Answer from the drawing. Dimensions are ordinates in mm from the lowest x, y and z of the part. Give positions to 0.01 mm unless a question says otherwise; leave off trailing zeros. Loops run counter-clockwise (first coordinate to the right, second up) from the corner with the lowest first, then second, coordinate; pieces in that order, holes last. Notation, with made-up numbers: M 46,9.25 L 89,9.25 A25 cw 89,40.25 Z; hole C 85,82.5 d10. An arc over 180 degrees is marked long. Use a Markdown table: item, result.
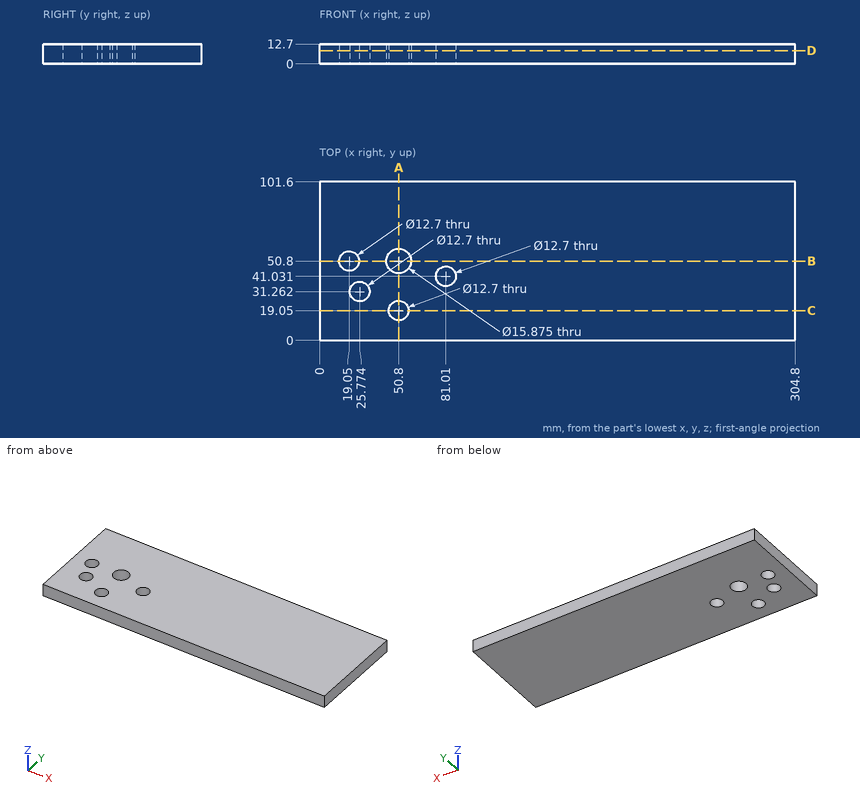
(1) A cutting plane is placed at A-A (x = 50.8). Write down the section's boundary in (y, z).
Entries:
| item | result |
|---|---|
| outline | M 0,0 L 12.7,0 L 12.7,12.7 L 0,12.7 Z; M 25.4,0 L 42.86,0 L 42.86,12.7 L 25.4,12.7 Z; M 58.74,0 L 101.6,0 L 101.6,12.7 L 58.74,12.7 Z |
(2) A cutting plane is placed at B-B (y = 50.8). Write down the section's boundary in (x, z), and give its area (3 significant figures).
Entries:
| item | result |
|---|---|
| outline | M 0,0 L 12.7,0 L 12.7,12.7 L 0,12.7 Z; M 25.4,0 L 42.86,0 L 42.86,12.7 L 25.4,12.7 Z; M 58.74,0 L 304.8,0 L 304.8,12.7 L 58.74,12.7 Z |
| area | 3,510 mm² |
(3) Consider probe 1 along Y at (x, z) = (50.8, 3.5); probe 2 along X at (y, z) = (53, 11.75) (1 decimal); probe 3 along Y at (x, z) = (19.05, 4.75). Determine where each line is inside the solid, lowest interval first. Write a range as [from, to].
Entries:
| item | result |
|---|---|
| probe 1 | y = [0, 12.7], [25.4, 42.86], [58.74, 101.6] |
| probe 2 | x = [0, 13.1], [25, 43.2], [58.4, 304.8] |
| probe 3 | y = [0, 44.45], [57.15, 101.6] |
(4) A cutting plane is placed at D-D (z = 8.5). Count the separate pieces of the cut face and the enclosed holes in it, and give its area (3 significant figures).
Entries:
| item | result |
|---|---|
| separate pieces | 1 |
| enclosed holes | 5 |
| area | 30,300 mm² |
(5) A cutting plane is placed at C-C (y = 19.05). Write down the section's boundary in (x, z), and give its area (3 significant figures).
Entries:
| item | result |
|---|---|
| outline | M 0,0 L 44.45,0 L 44.45,12.7 L 0,12.7 Z; M 57.15,0 L 304.8,0 L 304.8,12.7 L 57.15,12.7 Z |
| area | 3,710 mm² |
(6) Given P1, Ø10, axis at x = 270, y = 79, coming from the -Z side, flat-ended and moving along its own axis, determine where the tip first touches the part or whether it passes through.
Entries:
| item | result |
|---|---|
| P1 | stops at z = 0 |
